Here's how the part is built. I have some questions about the finished solid (model axes, mm). Coordinates: 2 decimals unless noted, no trailing zeros. Put each result on its own line as item: value. Start each with the question number.
Item 1: I need wall thicknesses on line 1 (Y direction, x = 24.5, z = 2.1); line 2 (Y direction, x = 14.5, z = 2.15); line 3 (Y direction, x = -45, z = 0.75). Which ranges of each line are inside material? Lowest first, please. Write a range as [from, to].
Item 2: If we mould it in two halves opening along X, with no side actions, what happens to faces 1 (the face through (25.2, 24.8, 1.5)), 2 (the face through (-1, 1, 3))? For each: released by +X, released by -X, zero draft, split by the parting line, or undercut.
Item 3: For pin 1 (0.9 mm diameter, centred on y = 46.5, z = 1.5, fed in from +X); pin 2 (1.5 mm diameter, centred on y = 48.5, z = 2, fed in from -X); pin 3 (0.9 mm diameter, centred on x = 88.5, z = 1, fed in from -Y), each with a flat end and sliding along its axis, tell me the tip position at first contact or that it passes through.
Item 4: I want a section at A-A, the plane z = 1.4. State how many separate pieces and enclosed holes the cut face has, then the cut area to 3 significant figures.
from build123d import *

# Parameters (mm, degrees)
EXTRUDE_1_DEPTH     = 3
HOLE_WIZARD_M31_D   = 3.2
SKETCH_6_W          = 6.5
SKETCH_6_H          = 7
CUT_EXTRUDE_1_DEPTH = 106.670478375
SKETCH_7_W          = 93
SKETCH_7_H          = 1.5
CUT_EXTRUDE_2_DEPTH = 106.670478375


with BuildPart() as part:
    # Эскиз1 → Бобышка-Вытянуть1 (new body)
    with BuildSketch(Plane.XY):
        with BuildLine():
            Line((92.5, -51), (92.5, -48.698957881))
            ThreePointArc((92.5, -48.698957881), (86.75, -47.5), (92.5, -46.301042119))
            Line((92.5, -46.301042119), (92.5, 46.301042119))
            ThreePointArc((92.5, 46.301042119), (86.75, 47.5), (92.5, 48.698957881))
            Line((92.5, 48.698957881), (92.5, 51))
            Line((92.5, 51), (-92.5, 51))
            Line((-92.5, 51), (-92.5, 48.698957881))
            ThreePointArc((-92.5, 48.698957881), (-86.75, 47.5), (-92.5, 46.301042119))
            Line((-92.5, 46.301042119), (-92.5, -46.301042119))
            ThreePointArc((-92.5, -46.301042119), (-86.75, -47.5), (-92.5, -48.698957881))
            Line((-92.5, -48.698957881), (-92.5, -51))
            Line((-92.5, -51), (92.5, -51))
        make_face()
    extrude(amount=EXTRUDE_1_DEPTH)

    # Отверстие с зазором M31 (through all)
    with Locations(Plane(origin=(0, 0, 0), x_dir=(-1, 0, 0), z_dir=(0, 0, -1))):
        with Locations((-76.53, -6.8), (-24.46, -1.72), (-24.46, 26.22), (-75.26, 41.46), (-69.63631327, -47.68571173), (-69.63631327, -10.94391141), (-32.25681239, -10.94391141), (-32.25681239, -47.68571173), (-14.5, 1), (53, 1), (3.25, 37), (69.75, 37)):
            Hole(HOLE_WIZARD_M31_D / 2)

    # Эскиз6 → Вырез-Вытянуть1 (cut, through all)
    with BuildSketch(Plane(origin=(0, 0, 0), x_dir=(-1, 0, 0), z_dir=(0, 0, -1))):
        with Locations((-89.75, 47.5)):
            Rectangle(SKETCH_6_W, SKETCH_6_H)
        with Locations((89.75, 47.5)):
            Rectangle(SKETCH_6_W, SKETCH_6_H)
        with Locations((89.75, -47.5)):
            Rectangle(SKETCH_6_W, SKETCH_6_H)
        with Locations((-89.75, -47.5)):
            Rectangle(SKETCH_6_W, SKETCH_6_H)
    extrude(amount=-CUT_EXTRUDE_1_DEPTH, mode=Mode.SUBTRACT)

    # Эскиз7 → Вырез-Вытянуть2 (cut, through all)
    with BuildSketch(Plane(origin=(0, 0, 0), x_dir=(-1, 0, 0), z_dir=(0, 0, -1))):
        with Locations((0, 50.25)):
            Rectangle(SKETCH_7_W, SKETCH_7_H)
    extrude(amount=-CUT_EXTRUDE_2_DEPTH, mode=Mode.SUBTRACT)


solid = part.part
Calculated:
1. line 1: y = [-51, -3.32], [-0.12, 24.62], [27.82, 49.5]
1. line 2: y = [-51, -0.6], [2.6, 49.5]
1. line 3: y = [-51, 49.5]
2. face 1: undercut
2. face 2: zero draft
3. pin 1: stops at x = 86.5
3. pin 2: stops at x = -86.5
3. pin 3: stops at y = -44
4. separate pieces: 1
4. enclosed holes: 12
4. area: 18,500 mm2
